CAD build for the part. Positions are in the model's coordinates, mm. Face numbers are marked on the shaded views. Coordinates: 2 decimals unless noted, no trailing zeros. Loops run counter-clockwise (first coordinate to the right, second up) from the corner with the lowest first, then second, coordinate; pieces in that order, holes last. Notation, with made-up numbers: (-33, -25.5) -> (-5, -25.5) arc R14 cw to (-5, -13.5) -> close; hole circle Ø7 at (-38, 9). An arc over 180 degrees is marked (long way). Return JSON: item names as keys, results as strings. Group by question number.
(1) Flat gauge pins, fed straight in: pin 1 Ø8 at (x, z) = (4.5, -4) entering from -Y; pin 2 Ø2 at (y, z) = (75, -12) entering from -X; pin 3 Ø10 at (x, y) = (-18.5, 104) entering from -Z; pin 4 Ø10 at (x, z) = (-20, -8.5) entering from -Y. Where does each tip first touch, or does it go through?
(2) Mould opens along X. For the marked faces 1, 2 and 3 say: pulls with the +X half, pulls with the -X half, needs draft (parallel to the pull), parting line crosses it, or undercut.
(3) Saw through at B-B on y = 133. Write the cut outline in (x, z), then the cut area to 3 significant figures.
(4) Probe L1, parallel to X at y = 140, z = 0; L2, parallel to Y at x = 14.5, z = -9; L3, parallel to Y at x = 0, z = 6.5. List the from-to ranges inside material, lowest first.
(5) Saw through at A-A on x = 0. Write the cut outline in (y, z), then the cut area to 3 significant figures.
(6) Saw through at C-C on z = 0. Write the cut outline in (x, y).
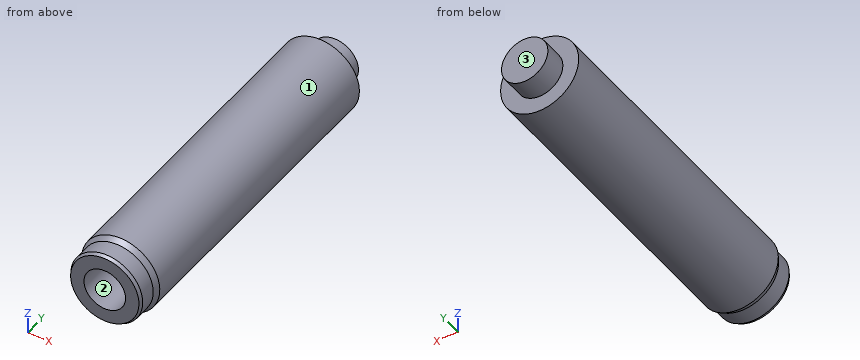
```python
from build123d import *

# Parameters (mm, degrees)
SKETCH1_R           = 25.25
SKETCH1_R_2         = 13.45
BOSS_EXTRUDE1_DEPTH = 216
SKETCH2_OUTSIDE_W   = 98
SKETCH2_OUTSIDE_H   = 98
SKETCH2_OUTSIDE_R   = 23.25
CUT_EXTRUDE1_DEPTH  = 12
CHAMFER2_SIZE       = 4
CHAMFER2_SIZE_2     = 2.309401077
CHAMFER3_SIZE       = 2
CHAMFER3_SIZE2      = 1.154700538
SKETCH3_R           = 15
INSIDE_HEAD_DEPTH   = 15


with BuildPart() as part:
    # Sketch1 → Boss-Extrude1 (new body)
    with BuildSketch(Plane(origin=(0, 0, 0), x_dir=(1, 0, 0), z_dir=(0, 1, 0))):
        with Locations(Location((0, 0, 0), (0, 0, 270))):
            Circle(SKETCH1_R)
        with Locations(Location((0, 0, 0), (0, 0, 270))):
            Circle(SKETCH1_R_2, mode=Mode.SUBTRACT)
    extrude(amount=BOSS_EXTRUDE1_DEPTH)

    # Sketch2 outside → Cut-Extrude1 (cut)
    with BuildSketch(Plane.XZ):
        Rectangle(SKETCH2_OUTSIDE_W, SKETCH2_OUTSIDE_H)
        with Locations(Location((0, 0, 0), (0, 0, 270))):
            Circle(SKETCH2_OUTSIDE_R, mode=Mode.SUBTRACT)
    extrude(amount=-CUT_EXTRUDE1_DEPTH, mode=Mode.SUBTRACT)

    # Chamfer2
    # the kernel refuses this chamfer: 4, 2.309401077 mm, written as the material it takes off along each edge
    with BuildSketch(Plane(origin=(0, 12, 0), x_dir=(0, 0, 1), z_dir=(1, 0, 0))) as chamfer2_piece_1_section:
        Polygon((25.25, -CHAMFER2_SIZE), (25.25 - CHAMFER2_SIZE_2, 0), (25.25, 0), align=None)
    chamfer2_piece_1 = revolve(axis=Axis((0, 12, 0), (0, -1, 0)), mode=Mode.PRIVATE)
    chamfer2_piece_1 = chamfer2_piece_1 - Plane(origin=(0, 14.291094123, 0), x_dir=(0, 0, -1), z_dir=(0, -1, 0)) * Cylinder(23.25, 101, mode=Mode.PRIVATE)
    add(chamfer2_piece_1, mode=Mode.SUBTRACT)

    # Chamfer3
    chamfer3_edges = [part.edges().sort_by_distance(p)[0] for p in [
        (0, 0, 23.25),
    ]]
    chamfer3_side = [part.faces().sort_by_distance(p)[0] for p in [
        (0, 6.267949193, 23.25),
    ]]
    chamfer(chamfer3_edges, length=CHAMFER3_SIZE, length2=CHAMFER3_SIZE2, reference=chamfer3_side[0])

    # Sketch3 → inside_head (add)
    with BuildSketch(Plane(origin=(0, 216, 0), x_dir=(1, 0, 0), z_dir=(0, 1, 0))):
        with Locations(Location((0, 0, 0), (0, 0, 270))):
            Circle(SKETCH3_R)
    extrude(amount=INSIDE_HEAD_DEPTH)


solid = part.part
```
Geometry results:
{
 "1": {"pin 1": "y = 216", "pin 2": "x = -22.73", "pin 3": "z = -21.34", "pin 4": "y = 0"},
 "2": {"face 1": "parting line crosses it", "face 2": "undercut", "face 3": "needs draft"},
 "3": {"outline": "circle Ø50.5 at (0, 0); hole circle Ø26.9 at (0, 0)", "area": "1,430 mm²"},
 "4": {"L1": "-25.25 to -13.45, 13.45 to 25.25", "L2": "0 to 216", "L3": "216 to 231"},
 "5": {"outline": "(0, -22.1) -> (2, -23.25) -> (12.54, -23.25) -> (16, -25.25) -> (216, -25.25) -> (216, -15) -> (231, -15) -> (231, 15) -> (216, 15) -> (216, 25.25) -> (16, 25.25) -> (12.54, 23.25) -> (2, 23.25) -> (0, 22.1) -> (0, 13.45) -> (216, 13.45) -> (216, -13.45) -> (0, -13.45) -> close", "area": "5,490 mm²"},
 "6": {"outline": "(-25.25, 16) -> (-23.25, 12.54) -> (-23.25, 2) -> (-22.1, 0) -> (-13.45, 0) -> (-13.45, 216) -> (13.45, 216) -> (13.45, 0) -> (22.1, 0) -> (23.25, 2) -> (23.25, 12.54) -> (25.25, 16) -> (25.25, 216) -> (15, 216) -> (15, 231) -> (-15, 231) -> (-15, 216) -> (-25.25, 216) -> close"}
}
